Work out the finished part from the listing and answer in its coordinate system (mm). Face numbers are marked on the shaded views. A direction names the side the tool comes from. Coordinates: 2 decimals unless noted, no trailing zeros. Order: outer loops, then holes, each group sorted by start corner. A loop starts at its lowest first (then second) coordinate and runs counter-clockwise, first axis right, second up.
```python
from build123d import *

# Parameters (mm, degrees)
SKETCH1_R            = 150
BOSS_EXTRUDE1_DEPTH  = 75
CHAMFER1_SIZE        = 10
BOSS_EXTRUDE2_START  = -75
BOSS_EXTRUDE2_DEPTH  = 10
CHAMFER2_SIZE        = 7
BOSS_EXTRUDE3_DEPTH  = 10
SKETCH7_R            = 4
CUT_EXTRUDE1_DEPTH   = 255.641782801
BOSS_EXTRUDE4_START  = 0.1
BOSS_EXTRUDE4_DEPTH  = 0.1
BOSS_EXTRUDE8_START  = -75
BOSS_EXTRUDE8_DEPTH  = 10
CHAMFER3_SIZE        = 7
BOSS_EXTRUDE9_DEPTH  = 10
SKETCH16_R           = 4
CUT_EXTRUDE2_DEPTH   = 302.407894506
CHAMFER4_SIZE        = 7
BOSS_EXTRUDE10_DEPTH = 10
SKETCH19_R           = 4
CUT_EXTRUDE3_DEPTH   = 302.407894506
BOSS_EXTRUDE11_START = -75
BOSS_EXTRUDE11_DEPTH = 10
CHAMFER5_SIZE        = 7
BOSS_EXTRUDE12_DEPTH = 10
SKETCH22_R           = 4
CUT_EXTRUDE4_DEPTH   = 302.407894506
CUT_EXTRUDE5_START   = -60
CUT_EXTRUDE5_DEPTH   = 60
CIRPATTERN31_COUNT   = 4
SKETCH24_R           = 110
BOSS_EXTRUDE13_DEPTH = 9
BOSS_EXTRUDE13_TAPER = 45
SKETCH25_R           = 10
BOSS_EXTRUDE14_DEPTH = 20
SKETCH28_R           = 4
CUT_EXTRUDE6_DEPTH   = 309.962325973


with BuildPart() as part:
    # Sketch1 → Boss-Extrude1 (new body)
    with BuildSketch(Plane(origin=(0, 0, 0), x_dir=(1, 0, 0), z_dir=(0, 1, 0))):
        with Locations(Location((0, 0, 0), (0, 0, 270))):
            Circle(SKETCH1_R)
    extrude(amount=BOSS_EXTRUDE1_DEPTH)

    # Chamfer1
    chamfer1_edges = [part.edges().sort_by_distance(p)[0] for p in [
        (0, 75, -150),
    ]]
    chamfer(chamfer1_edges, length=CHAMFER1_SIZE)

    # Sketch2 → Boss-Extrude2 (add)
    with BuildSketch(Plane(origin=(0, 75, 0), x_dir=(1, 0, 0), z_dir=(0, 1, 0)).offset(BOSS_EXTRUDE2_START)):
        with BuildLine():
            Line((-145.236875483, 37.5), (-195.236875483, 37.5))
            Line((-195.236875483, 37.5), (-195.236875483, -37.5))
            Line((-195.236875483, -37.5), (-145.236875483, -37.5))
            ThreePointArc((-145.236875483, -37.5), (-150, 0), (-145.236875483, 37.5))
        make_face()
    extrude(amount=BOSS_EXTRUDE2_DEPTH)

    # Chamfer2
    chamfer2_edges = [part.edges().sort_by_distance(p)[0] for p in [
        (-195.236875483, 5, 37.5),
        (-195.236875483, 5, -37.5),
    ]]
    chamfer(chamfer2_edges, length=CHAMFER2_SIZE)

    # Sketch6 → Boss-Extrude3 (add)
    with BuildSketch(Plane.XY.offset(37.5)):
        Polygon((-145.236875483, 0), (-145.236875483, 65), (-170.556875483, 65), (-188.236875483, 10), (-188.236875483, 0), align=None)
    boss_extrude3 = extrude(amount=-BOSS_EXTRUDE3_DEPTH)

    # Sketch7 → Cut-Extrude1 (cut, through all)
    with BuildSketch(Plane(origin=(0, 10, 0), x_dir=(1, 0, 0), z_dir=(0, 1, 0))):
        with Locations(Location((-172.618437741, -13.75, 0), (0, 0, 270))):
            Circle(SKETCH7_R)
    cut_extrude1 = extrude(amount=-CUT_EXTRUDE1_DEPTH, mode=Mode.SUBTRACT)

    # Mirror2: Boss-Extrude3, Cut-Extrude1 across plane
    add(boss_extrude3.mirror(Plane.XY))
    add(cut_extrude1.mirror(Plane.XY), mode=Mode.SUBTRACT)

    # Sketch10 → Boss-Extrude4 (add)
    with BuildSketch(Plane.XZ.offset(BOSS_EXTRUDE4_START)):
        with BuildLine():
            Line((-145.236875483, 37.5), (-188.236875483, 37.5))
            Line((-188.236875483, 37.5), (-195.236875483, 30.5))
            Line((-195.236875483, 30.5), (-195.236875483, -30.5))
            Line((-195.236875483, -30.5), (-188.236875483, -37.5))
            Line((-188.236875483, -37.5), (-145.236875483, -37.5))
            ThreePointArc((-145.236875483, -37.5), (-150, 0), (-145.236875483, 37.5))
        make_face()
    extrude(amount=-BOSS_EXTRUDE4_DEPTH)

    # Sketch11 → Boss-Extrude8 (add)
    with BuildSketch(Plane(origin=(0, 75, 0), x_dir=(1, 0, 0), z_dir=(0, 1, 0)).offset(BOSS_EXTRUDE8_START)):
        with BuildLine():
            Line((37.5, 220.236875483), (37.5, 145.236875483))
            ThreePointArc((37.5, 145.236875483), (0, 150), (-37.5, 145.236875483))
            Line((-37.5, 145.236875483), (-37.5, 220.236875483))
            Line((-37.5, 220.236875483), (37.5, 220.236875483))
        make_face()
        with BuildLine():
            Line((37.5, -220.236875483), (37.5, -145.236875483))
            ThreePointArc((37.5, -145.236875483), (0, -150), (-37.5, -145.236875483))
            Line((-37.5, -145.236875483), (-37.5, -220.236875483))
            Line((-37.5, -220.236875483), (37.5, -220.236875483))
        make_face()
    extrude(amount=BOSS_EXTRUDE8_DEPTH)

    # Chamfer3
    chamfer3_edges = [part.edges().sort_by_distance(p)[0] for p in [
        (37.5, 5, -220.236875483),
        (-37.5, 5, -220.236875483),
    ]]
    chamfer(chamfer3_edges, length=CHAMFER3_SIZE)

    # Sketch14 → Boss-Extrude9 (add)
    with BuildSketch(Plane.ZY.offset(37.5)):
        Polygon((-145.236875483, 0), (-145.236875483, 65), (-195.556875483, 65), (-213.236875483, 10), (-213.236875483, 0), align=None)
    boss_extrude9 = extrude(amount=-BOSS_EXTRUDE9_DEPTH)

    # Mirror3: Boss-Extrude9 across plane
    add(boss_extrude9.mirror(Plane.ZY))

    # Sketch16 → Cut-Extrude2 (cut, through all)
    with BuildSketch(Plane(origin=(0, 10, 0), x_dir=(1, 0, 0), z_dir=(0, 1, 0))):
        with Locations(Location((-13.75, 185.118437741, 0), (0, 0, 270))):
            Circle(SKETCH16_R)
        with Locations(Location((13.75, 185.118437741, 0), (0, 0, 270))):
            Circle(SKETCH16_R)
    extrude(amount=-CUT_EXTRUDE2_DEPTH, mode=Mode.SUBTRACT)

    # Chamfer4
    chamfer4_edges = [part.edges().sort_by_distance(p)[0] for p in [
        (-37.5, 5, 220.236875483),
        (37.5, 5, 220.236875483),
    ]]
    chamfer(chamfer4_edges, length=CHAMFER4_SIZE)

    # Sketch18 → Boss-Extrude10 (add)
    with BuildSketch(Plane(origin=(37.5, 0, 0), x_dir=(0, 0, -1), z_dir=(1, 0, 0))):
        Polygon((-145.236875483, 0), (-145.236875483, 65), (-196.456875483, 65), (-213.236875483, 10), (-213.236875483, 0), align=None)
    boss_extrude10 = extrude(amount=-BOSS_EXTRUDE10_DEPTH)

    # Sketch19 → Cut-Extrude3 (cut, through all)
    with BuildSketch(Plane(origin=(0, 10, 0), x_dir=(1, 0, 0), z_dir=(0, 1, 0))):
        with Locations(Location((13.75, -184.771281751, 0), (0, 0, 270))):
            Circle(SKETCH19_R)
        with Locations(Location((-13.75, -184.771281751, 0), (0, 0, 270))):
            Circle(SKETCH19_R)
    extrude(amount=-CUT_EXTRUDE3_DEPTH, mode=Mode.SUBTRACT)

    # Mirror4: Boss-Extrude10 across plane
    add(boss_extrude10.mirror(Plane(origin=(0, 0, 0), x_dir=(0, 0, 1), z_dir=(1, 0, 0))))

    # Sketch20 → Boss-Extrude11 (add)
    with BuildSketch(Plane(origin=(0, 75, 0), x_dir=(1, 0, 0), z_dir=(0, 1, 0)).offset(BOSS_EXTRUDE11_START)):
        with BuildLine():
            Line((195.236875483, 37.5), (145.236875483, 37.5))
            ThreePointArc((145.236875483, 37.5), (150, 0), (145.236875483, -37.5))
            Line((145.236875483, -37.5), (195.236875483, -37.5))
            Line((195.236875483, -37.5), (195.236875483, 37.5))
        make_face()
    extrude(amount=BOSS_EXTRUDE11_DEPTH)

    # Chamfer5
    chamfer5_edges = [part.edges().sort_by_distance(p)[0] for p in [
        (195.236875483, 5, 37.5),
        (195.236875483, 5, -37.5),
    ]]
    chamfer(chamfer5_edges, length=CHAMFER5_SIZE)

    # Sketch21 → Boss-Extrude12 (add)
    with BuildSketch(Plane(origin=(0, 0, -37.5), x_dir=(-1, 0, 0), z_dir=(0, 0, -1))):
        Polygon((-145.236875483, 0), (-145.236875483, 65), (-170.556875483, 65), (-188.236875483, 10), (-188.236875483, 0), align=None)
    boss_extrude12 = extrude(amount=-BOSS_EXTRUDE12_DEPTH)

    # Sketch22 → Cut-Extrude4 (cut, through all)
    with BuildSketch(Plane(origin=(0, 10, 0), x_dir=(1, 0, 0), z_dir=(0, 1, 0))):
        with Locations(Location((172.618437741, 13.75, 0), (0, 0, 270))):
            Circle(SKETCH22_R)
    cut_extrude4 = extrude(amount=-CUT_EXTRUDE4_DEPTH, mode=Mode.SUBTRACT)

    # Mirror5: Boss-Extrude12, Cut-Extrude4 across plane
    add(boss_extrude12.mirror(Plane(origin=(0, 0, 0), x_dir=(1, 0, 0), z_dir=(0, 0, -1))))
    add(cut_extrude4.mirror(Plane(origin=(0, 0, 0), x_dir=(1, 0, 0), z_dir=(0, 0, -1))), mode=Mode.SUBTRACT)

    # Sketch23 → Cut-Extrude5 (cut)
    with BuildSketch(Plane(origin=(0, 75, 0), x_dir=(1, 0, 0), z_dir=(0, 1, 0)).offset(CUT_EXTRUDE5_START)):
        with BuildLine():
            Line((-103.923048454, -60), (-129.903810568, -75))
            ThreePointArc((-129.903810568, -75), (-106.066017178, -106.066017178), (-75, -129.903810568))
            Line((-75, -129.903810568), (-60, -103.923048454))
            ThreePointArc((-60, -103.923048454), (-84.852813742, -84.852813742), (-103.923048454, -60))
        make_face()
    cut_extrude5 = extrude(amount=CUT_EXTRUDE5_DEPTH, mode=Mode.SUBTRACT)

    # CirPattern31: Cut-Extrude5 ×4 about axis
    cirpattern31_axis = Axis((0, 75, 0), (0, 1, 0))
    for i in range(1, CIRPATTERN31_COUNT):
        add(cut_extrude5.rotate(cirpattern31_axis, i * 360 / CIRPATTERN31_COUNT), mode=Mode.SUBTRACT)

    # Sketch24 → Boss-Extrude13 (add)
    with BuildSketch(Plane(origin=(0, 75, 0), x_dir=(1, 0, 0), z_dir=(0, 1, 0))):
        Circle(SKETCH24_R)
    extrude(amount=BOSS_EXTRUDE13_DEPTH, taper=BOSS_EXTRUDE13_TAPER)

    # Sketch25 → Boss-Extrude14 (add)
    with BuildSketch(Plane(origin=(0, 84, 0), x_dir=(1, 0, 0), z_dir=(0, 1, 0))):
        with Locations(Location((0, 0, 0), (0, 0, 270))):
            Circle(SKETCH25_R)
    extrude(amount=BOSS_EXTRUDE14_DEPTH)

    # Sketch28 → Cut-Extrude6 (cut, through all)
    with BuildSketch(Plane(origin=(0, 10, 0), x_dir=(1, 0, 0), z_dir=(0, 1, 0))):
        with Locations(Location((-172.618437741, 13.75, 0), (0, 0, 270))):
            Circle(SKETCH28_R)
        with Locations(Location((-172.618437741, -13.75, 0), (0, 0, 270))):
            Circle(SKETCH28_R)
    extrude(amount=-CUT_EXTRUDE6_DEPTH, mode=Mode.SUBTRACT)


solid = part.part
```
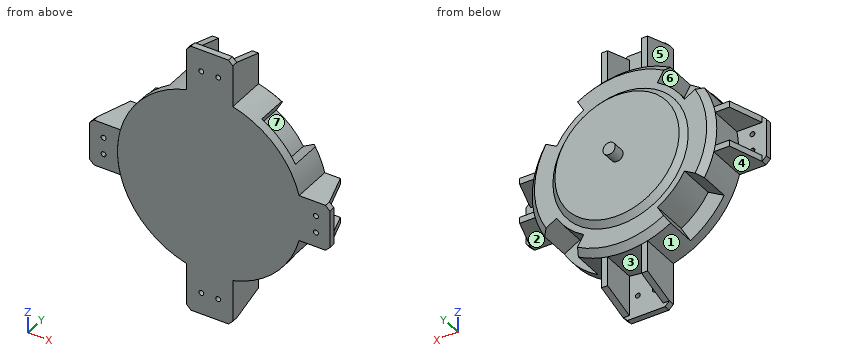
1. Consider probe 1 along X at (y, z) = (0.05, 13.75); probe 2 along X at (y, z) = (52.5, 189); probe 3 along Z at (x, y) = (60.5, 25). Determine where each line is inside the solid, lowest interval first.
2. The mould has two halves that part along X. Classify the marked faces 1, 2 and 3: released by +X, released by -X, zero draft, split by the parting line, or undercut.
3. The part is cut by section B-B (y = 98). Determine the outline of the cut face in (x, z).
4. The part is cut by section A-A (x = -158.5). Determine the outline of the cut face in (y, z), plus the area to 3 significant figures.
5. For the marked faces 4, 5, 6 and 7, determine the directions among +Z, -Z, +X, -X, +Y, -Y from which every point of the face is accessible in a straight line to the end or side of a thin tool.
6. Flat-ended cylindrical pins translate along their axes: pin 1 (2 mm diameter, centred on x = -69.5, y = 83, fed in from -Z); pin 2 (10 mm diameter, centred on y = 81.5, z = 14.5, fed in from -X); pin 3 (8 mm diameter, centred on y = 77.5, z = 75, fed in from -X). Find the tip coordinate at first contact, or state that the pin passes through.
Worked out:
1. probe 1: x = -195.24 to -176.62, -168.62 to 168.62, 176.62 to 195.24
1. probe 2: x = -37.5 to -27.5, 27.5 to 37.5
1. probe 3: z = -137.26 to -104.79, -103.63 to 103.63, 104.79 to 137.26
2. face 1: released by -X
2. face 2: zero draft
2. face 3: undercut
3. outline: circle Ø20 at (0, 0)
4. outline: (-0.1, -37.5) - (65, -37.5) - (65, -27.5) - (10, -27.5) - (10, 27.5) - (65, 27.5) - (65, 37.5) - (-0.1, 37.5) - close
4. area: 1,860 mm2
5. face 4: -Z, -X, +Y, -Y
5. face 5: +Z, -X, +Y, -Y
5. face 6: -X, +Y
5. face 7: +Y
6. pin 1: stops at z = -76.3
6. pin 2: stops at x = -107.57
6. pin 3: stops at x = -96.09
